```python
from build123d import *

# Parameters (mm, degrees)
SKETCH_1_W          = 140
SKETCH_1_H          = 72
SKETCH_1_R          = 1.6
SKETCH_1_R_2        = 4
EXTRUDE_1_DEPTH     = 5
SKETCH_2_W          = 29
SKETCH_2_H          = 21
SKETCH_2_W_2        = 46
SKETCH_2_H_2        = 19
CUT_EXTRUDE_1_DEPTH = 79.873316147
FILLET_1_R          = 3
CHAMFER_1_SIZE      = 8


with BuildPart() as part:
    # 草图1 → 凸台-拉伸1 (new body)
    with BuildSketch(Plane.XY):
        Rectangle(SKETCH_1_W, SKETCH_1_H)
        with Locations((-25, 6)):
            Circle(SKETCH_1_R, mode=Mode.SUBTRACT)
        with Locations((25, 6)):
            Circle(SKETCH_1_R, mode=Mode.SUBTRACT)
        with Locations((-25, -6)):
            Circle(SKETCH_1_R, mode=Mode.SUBTRACT)
        with Locations((25, -6)):
            Circle(SKETCH_1_R, mode=Mode.SUBTRACT)
        Circle(SKETCH_1_R_2, mode=Mode.SUBTRACT)
    extrude(amount=EXTRUDE_1_DEPTH)

    # 草图2 → 切除-拉伸1 (cut, through all)
    with BuildSketch(Plane.XY.offset(5)):
        with Locations((-47.5, 15.5)):
            Rectangle(SKETCH_2_W, SKETCH_2_H)
        with Locations((-47.5, -15.5)):
            Rectangle(SKETCH_2_W, SKETCH_2_H)
        with Locations((47.5, -15.5)):
            Rectangle(SKETCH_2_W, SKETCH_2_H)
        with Locations((47.5, 15.5)):
            Rectangle(SKETCH_2_W, SKETCH_2_H)
        with Locations((0, 18.5)):
            Rectangle(SKETCH_2_W_2, SKETCH_2_H_2)
        with Locations((0, -18.5)):
            Rectangle(SKETCH_2_W_2, SKETCH_2_H_2)
    extrude(amount=-CUT_EXTRUDE_1_DEPTH, mode=Mode.SUBTRACT)

    # 圆角1
    fillet_1_edges = [part.edges().sort_by_distance(p)[0] for p in [
        (-62, -26, 2.5),
        (-62, -5, 2.5),
        (-33, -5, 2.5),
        (-33, -26, 2.5),
        (23, 28, 2.5),
        (23, 9, 2.5),
        (-23, 9, 2.5),
        (-23, 28, 2.5),
        (62, -5, 2.5),
        (62, -26, 2.5),
        (33, -26, 2.5),
        (33, -5, 2.5),
        (62, 26, 2.5),
        (62, 5, 2.5),
        (33, 5, 2.5),
        (33, 26, 2.5),
        (23, -9, 2.5),
        (23, -28, 2.5),
        (-23, -28, 2.5),
        (-23, -9, 2.5),
        (-62, 5, 2.5),
        (-62, 26, 2.5),
        (-33, 26, 2.5),
        (-33, 5, 2.5),
    ]]
    fillet(fillet_1_edges, radius=FILLET_1_R)

    # 倒角1
    chamfer_1_edges = [part.edges().sort_by_distance(p)[0] for p in [
        (-70, 36, 2.5),
        (70, 36, 2.5),
        (70, -36, 2.5),
        (-70, -36, 2.5),
    ]]
    chamfer(chamfer_1_edges, length=CHAMFER_1_SIZE)


solid = part.part
```
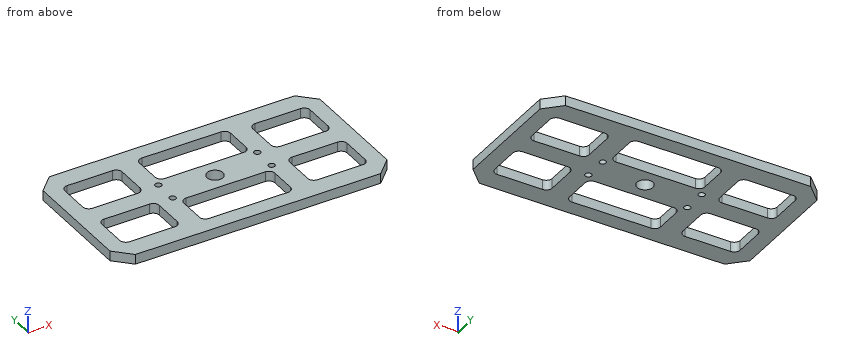
Design review of the part built by this model. Coordinates are the model's own, in mm. Coordinates: 2 decimals unless noted, no trailing zeros. Order: outer loops, then holes, each group sorted by start corner. A loop starts at its lowest first (then second) coordinate and runs counter-clockwise, first axis right, second up.
1) Take a section at C-C, the plane x = 14. Give the boundary of the cut face in (y, z).
2) Take a section at D-D, the plane x = -48.5. Give the boundary of the cut face in (y, z), and give its area (3 significant figures).
3) Wall thickness on line 1 along Y through (x, z) = (25, 2.9); line 2 along Y through (x, z) = (-44, 1.85); line 3 along X through (y, z) = (19, 3.8): over which ranges is each line inside the solid? List them lowest first.
4) Take a section at B-B, the plane x = 0. Give the boundary of the cut face in (y, z).
5) Take a section at A-A, the plane y = -21.5. Give the boundary of the cut face in (x, z), and give its area (3 significant figures).
Returned:
1. outline: (-36, 0) - (-28, 0) - (-28, 5) - (-36, 5) - close; (-9, 0) - (9, 0) - (9, 5) - (-9, 5) - close; (28, 0) - (36, 0) - (36, 5) - (28, 5) - close
2. outline: (-36, 0) - (-26, 0) - (-26, 5) - (-36, 5) - close; (-5, 0) - (5, 0) - (5, 5) - (-5, 5) - close; (26, 0) - (36, 0) - (36, 5) - (26, 5) - close
2. area: 150 mm2
3. line 1: y = -36 to -7.6, -4.4 to 4.4, 7.6 to 36
3. line 2: y = -36 to -26, -5 to 5, 26 to 36
3. line 3: x = -70 to -62, -33 to -23, 23 to 33, 62 to 70
4. outline: (-36, 0) - (-28, 0) - (-28, 5) - (-36, 5) - close; (-9, 0) - (-4, 0) - (-4, 5) - (-9, 5) - close; (4, 0) - (9, 0) - (9, 5) - (4, 5) - close; (28, 0) - (36, 0) - (36, 5) - (28, 5) - close
5. outline: (-70, 0) - (-62, 0) - (-62, 5) - (-70, 5) - close; (-33, 0) - (-23, 0) - (-23, 5) - (-33, 5) - close; (23, 0) - (33, 0) - (33, 5) - (23, 5) - close; (62, 0) - (70, 0) - (70, 5) - (62, 5) - close
5. area: 180 mm2
